```python
from build123d import *

# Parameters (mm, degrees)
CYLINDER005_R     = 1
CYLINDER005_DEPTH = 10
CYLINDER004_R     = 1
CYLINDER004_DEPTH = 10
CYLINDER001_R     = 2
CYLINDER001_DEPTH = 0.2
CYLINDER_R        = 2
CYLINDER_DEPTH    = 0.2
BOX008_W          = 8
BOX008_H          = 16
BOX008_DEPTH      = 0.2


with BuildPart() as cilindro005:
    # Cylinder005 → Cylinder005 (new body)
    with BuildSketch(Plane(origin=(38.5, 11, 1), x_dir=(1, 0, 0), z_dir=(0, 0, 1))):
        Circle(CYLINDER005_R)
    extrude(amount=CYLINDER005_DEPTH)


with BuildPart() as cilindro004:
    # Cylinder004 → Cylinder004 (new body)
    with BuildSketch(Plane(origin=(38.5, 27, 1), x_dir=(1, 0, 0), z_dir=(0, 0, 1))):
        Circle(CYLINDER004_R)
    extrude(amount=CYLINDER004_DEPTH)


with BuildPart() as cilindro001:
    # Cylinder001 → Cylinder001 (new body)
    with BuildSketch(Plane(origin=(39, 26.5, 1), x_dir=(1, 0, 0), z_dir=(0, 0, 1))):
        Circle(CYLINDER001_R)
    extrude(amount=CYLINDER001_DEPTH)


with BuildPart() as cilindro:
    # Cylinder → Cylinder (new body)
    with BuildSketch(Plane(origin=(39, 10.5, 1), x_dir=(1, 0, 0), z_dir=(0, 0, 1))):
        Circle(CYLINDER_R)
    extrude(amount=CYLINDER_DEPTH)


with BuildPart() as obj1:
    # Box008 → Box008 (new body)
    with BuildSketch(Plane(origin=(35, 10.5, 1), x_dir=(1, 0, 0), z_dir=(0, 0, 1))):
        with Locations((4, 8)):
            Rectangle(BOX008_W, BOX008_H)
    extrude(amount=BOX008_DEPTH)

    # Fusion: union Cilindro001, Cilindro
    add(cilindro001.part)
    add(cilindro.part)


with BuildPart() as obj1_1:
    # Fusion placement: moved
    add(obj1.part.moved(Location((-0.5, 0.5, 4.8))))

    # Cut005: cut Cilindro004
    add(cilindro004.part, mode=Mode.SUBTRACT)

    # Cut006: cut Cilindro005
    add(cilindro005.part, mode=Mode.SUBTRACT)


solid = obj1_1.part
```
Geometry check sheet. Reference: the model listing, model coordinates, mm. Round coordinates to 2 decimals unless told otherwise and drop trailing zeros. Order: outer loops, then holes, each group sorted by start corner. A loop starts at its lowest first (then second) coordinate and runs counter-clockwise, first axis right, second up. Notation, with made-up numbers: M 43.5,-40 L 60.5,-40 A32 ccw 60.5,-14 Z; hole C 21,-29.75 d7. An arc over 180 degrees is marked long. Answer as CSV lines item,"result".
1) Sectioned sample at C-C on x = 35.75. Record the cut outline in (y, z), and give its area (3 significant figures).
Entries:
outline,"M 11,5.8 L 27,5.8 L 27,6 L 11,6 Z"
area,"3.20 mm2"
2) Sectioned sample at A-A on x = 38.5. Record the cut outline in (y, z), and give its area (3 significant figures).
Entries:
outline,"M 9,5.8 L 10,5.8 L 10,6 L 9,6 Z; M 12,5.8 L 26,5.8 L 26,6 L 12,6 Z; M 28,5.8 L 29,5.8 L 29,6 L 28,6 Z"
area,"3.20 mm2"
3) Sectioned sample at B-B on z = 5.9. Record the cut outline in (x, y), and give its area (3 significant figures).
Entries:
outline,"M 34.5,11 L 36.5,11 A2 ccw 40.5,11 L 42.5,11 L 42.5,27 L 40.5,27 A2 ccw 36.5,27 L 34.5,27 Z; hole C 38.5,11 d2; hole C 38.5,27 d2"
area,"134 mm2"
4) Thickness scan on probe 1 along Y at (x, z) = (38.5, 5.9); probe 2 along Y at (x, z) = (39.25, 5.85); probe 3 along Y at (x, z) = (41.5, 5.85). Record the ranges inside material, lowest first. Write a range as [from, to].
Entries:
probe 1,"[9, 10], [12, 26], [28, 29]"
probe 2,"[9.15, 10.34], [11.66, 26.34], [27.66, 28.85]"
probe 3,"[11, 27]"
